Geometry: final body of the model. Coordinates: model frame, mm. Face numbers are marked on the shaded views. A direction names the side the tool comes from. Give positions to 0.01 mm unless a question says otherwise; leave off trailing zeros. Order: outer loops, then holes, each group sorted by start corner. A loop starts at its lowest first (then second) coordinate and runs counter-clockwise, first axis right, second up. Notation, with made-up numbers: (-27.5, 28) -> (8.5, 28) arc R10 ccw to (8.5, 40) -> close; hole circle Ø10 at (59, 57.25). An arc over 180 degrees is marked (long way). One line per item, written item: value. Start each with the question number.
```python
from build123d import *

# Parameters (mm, degrees)
F0_W     = 4.5
F0_H     = 1.1
F1_DEPTH = 0.6
F2_W     = 4.5
F2_H     = 2.2
F3_DEPTH = 1.6
F4_R     = 1.09999
F5_R     = 0.5
F6_DEPTH = 25


# Not quite as in the source:
# - a fillet or chamfer is up to 0.001 mm smaller than in the source, because OpenCascade refuses the exact size


with BuildPart() as f1:
    # F0 (on Top) → F1 (new body)
    with BuildSketch(Plane.XY):
        with Locations((12.05, 2.05)):
            Rectangle(F0_W, F0_H)
        with Locations((12.05, 3.15)):
            Rectangle(F0_W, F0_H)
        with BuildLine():
            Line((9.1267705413, 1.5), (9.8, 1.5))
            Line((9.8, 1.5), (9.8, 2.6))
            Line((9.8, 2.6), (8.8, 2.6))
            Line((8.8, 2.6), (8.8, 1.4793838437))
            ThreePointArc((8.8, 1.4793838437), (8.9630604221, 1.4948408423), (9.1267705413, 1.5))
        make_face()
        with BuildLine():
            Line((8.8, 2.6), (9.8, 2.6))
            Line((9.8, 2.6), (9.8, 3.7))
            Line((9.8, 3.7), (9.1267705413, 3.7))
            ThreePointArc((9.1267705413, 3.7), (8.9630604221, 3.7051591577), (8.8, 3.7206161563))
            Line((8.8, 3.7206161563), (8.8, 2.6))
        make_face()
        with BuildLine():
            Line((8.8, 1.4793838437), (8.8, 2.6))
            Line((8.8, 2.6), (8.8, 3.7206161563))
            ThreePointArc((8.8, 3.7206161563), (8.6407616767, 3.7458278477), (8.4833920771, 3.7808604342))
            Line((8.4833920771, 3.7808604342), (3.2433784641, 5.1191395658))
            ThreePointArc((3.2433784641, 5.1191395658), (2.9242199323, 5.1797056878), (2.6, 5.2))
            Line((2.6, 5.2), (2.6, 4.2))
            ThreePointArc((2.6, 4.2), (3.7313708499, 3.7313708499), (4.2, 2.6))
            ThreePointArc((4.2, 2.6), (3.7313708499, 1.4686291501), (2.6, 1))
            Line((2.6, 1), (2.6, 0))
            ThreePointArc((2.6, 0), (2.9242199323, 0.0202943122), (3.2433784641, 0.0808604342))
            Line((3.2433784641, 0.0808604342), (8.4833920771, 1.4191395658))
            ThreePointArc((8.4833920771, 1.4191395658), (8.6407616767, 1.4541721523), (8.8, 1.4793838437))
        make_face()
        with BuildLine():
            ThreePointArc((0, 2.6), (0.7615223689, 0.7615223689), (2.6, 0))
            Line((2.6, 0), (2.6, 1))
            ThreePointArc((2.6, 1), (1, 2.6), (2.6, 4.2))
            Line((2.6, 4.2), (2.6, 5.2))
            ThreePointArc((2.6, 5.2), (0.7615223689, 4.4384776311), (0, 2.6))
        make_face()
    extrude(amount=F1_DEPTH)

    # F2 (on face) → F3 (join)
    with BuildSketch(Plane.XY.offset(0.6)):
        with Locations((12.05, 2.6)):
            Rectangle(F2_W, F2_H)
    extrude(amount=F3_DEPTH)

    # F4 (radius 1.1 in the source; OpenCascade refuses exactly that, so slightly less here)
    f4_edges = [f1.edges().sort_by_distance(p)[0] for p in [
        (12.05, 1.5, 2.2),
        (12.05, 3.7, 2.2),
    ]]
    fillet(f4_edges, radius=F4_R)

    # F5 (on face) → F6 (cut)
    with BuildSketch(Plane.YZ.offset(14.3)):
        with Locations((2.6, 1.1)):
            Circle(F5_R)
    extrude(amount=-F6_DEPTH, mode=Mode.SUBTRACT)


solid = f1.part
```
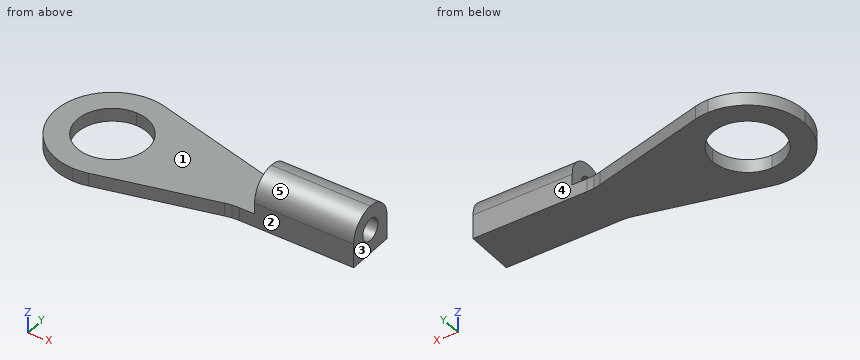
1. Cut plane C-C, the plane y = 3.5. Return loops of the section in (x, z), then the cut area to 3 significant figures.
2. Cut plane D-D, the plane x = 3.75. Return loops of the section in (y, z).
3. Cut plane B-B, the plane z = 1.45. Return loops of the section in (x, y).
4. Pin query (flat end, axial travel): P1, Ø3, axis at x = 5, y = 1, coming from the +Z side; P2, Ø1.2, axis at x = 12, z = 0.5, coming from the -Y side; P3, Ø0.5, axis at y = 2, z = 2, coming from the -X side. Return the tip coordinate at first contact, or that it passes through.
5. Access query for the marked faces 1, 2, 3, 4 and 5. Directions: +Z, -Z, +X, -X, +Y, -Y. A direction counts if a zero-diameter tool reaches every point of the face in a straight line with its end or side. Return the directions, or none.
6. Material intervals for L1, parallel to Z at x = 12.7, y = 2.6; L2, parallel to Y at x = 10.9, z = 1.1; L3, parallel to X at y = 2.9, z = 1.9, sorted ascending. Write a range as [from, to].
Answers follow:
1. outline: (0.16, 0) -> (1.28, 0) -> (1.28, 0.6) -> (0.16, 0.6) -> close; (3.92, 0) -> (14.3, 0) -> (14.3, 1.73) -> (9.8, 1.73) -> (9.8, 0.6) -> (3.92, 0.6) -> close
1. area: 12.0 mm²
2. outline: (0.21, 0) -> (1.49, 0) -> (1.49, 0.6) -> (0.21, 0.6) -> close; (3.71, 0) -> (4.99, 0) -> (4.99, 0.6) -> (3.71, 0.6) -> close
3. outline: (9.8, 1.56) -> (14.3, 1.56) -> (14.3, 2.24) -> (9.8, 2.24) -> close; (9.8, 2.96) -> (14.3, 2.96) -> (14.3, 3.64) -> (9.8, 3.64) -> close
4. P1: stops at z = 0.6
4. P2: stops at y = 1.5
4. P3: stops at x = 9.8
5. face 1: +Z, -X, +Y, -Y
5. face 2: +Z, -Z, +X, -Y
5. face 3: +Z, -Z, +X, +Y, -Y
5. face 4: +Z, -Z, +X, +Y
5. face 5: +Z, +X, -X, -Y
6. L1: z = [0, 0.6], [1.6, 2.2]
6. L2: y = [1.5, 2.1], [3.1, 3.7]
6. L3: x = [9.8, 14.3]
